Design review of the part built by this model. Coordinates are the model's own, in mm. Face numbers are marked on the shaded views. Coordinates: 2 decimals unless noted, no trailing zeros. Write each loop counter-clockwise with the first axis right and the second up, starting at its lowest first coordinate (ties: lowest second). Pieces come first, ordered by that corner, then holes. Notation, with made-up numbers: M -38.75,3.5 L -11.75,3.5 A20 ccw -11.75,13.5 Z; hole C -34.5,89.5 d8. An arc over 180 degrees is marked long. Write item = value, one per line.
```python
from build123d import *

# Parameters (mm, degrees)
F1_DEPTH = 53.975


with BuildPart() as f1:
    # F0 (on Right) → F1 (new body, symmetric)
    with BuildSketch(Plane.YZ):
        Polygon((-25.4, 14.664697), (-25.4, -14.664697), (0, -29.329394), (25.4, -14.664697), (25.4, 14.664697), (0, 29.329394), align=None)
    extrude(amount=F1_DEPTH, both=True)

    # F2 (on Front) → F3 (revolve, cut)
    with BuildSketch(Plane.XZ):
        Polygon((-53.975, 0), (53.975, 0), (53.975, 12.192), (-26.401746, 12.192), (-53.975, 20.543119), align=None)
    revolve(axis=Axis((-0.356656, 0, 0), (1, 0, 0)), mode=Mode.SUBTRACT)


solid = f1.part
```
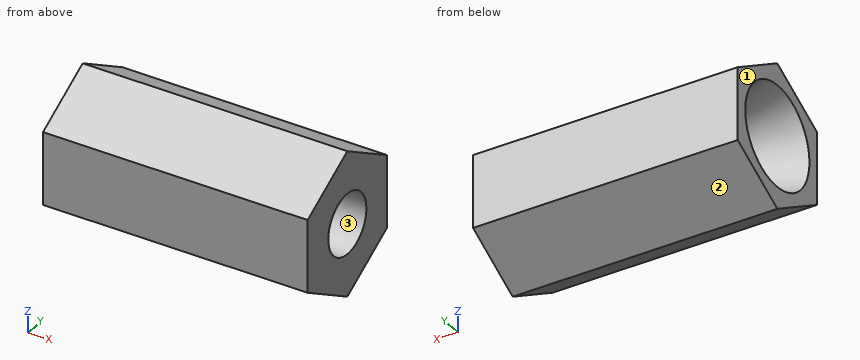
Q1. Consider section B-B, the plane z = 0. State the section outline as (x, y) points (3 decimals), and give its area (3 significant figures).
Check result:
outline = M -53.975,-25.4 L 53.975,-25.4 L 53.975,-12.192 L -26.402,-12.192 L -53.975,-20.543 Z; M -53.975,20.543 L -26.402,12.192 L 53.975,12.192 L 53.975,25.4 L -53.975,25.4 Z
area = 2,620 mm²
Q2. Consider section C-C, the plane z = -23.5. State the section outline as (x, y) points (3 decimals).
Check result:
outline = M -53.975,-10.097 L 53.975,-10.097 L 53.975,10.097 L -53.975,10.097 Z
Q3. Wall thickness on line 1 (Y direction, x = 25, z = 0); line 2 (Z direction, x = -9, y = 0); line 3 (Y direction, x = -37, z = -12): over which ranges is each line inside the solid? List them lowest first.
Check result:
line_1 = -25.4 to -12.19, 12.19 to 25.4
line_2 = -29.33 to -12.19, 12.19 to 29.33
line_3 = -25.4 to -9.65, 9.65 to 25.4
Q4. Consider section A-A, the plane x = 46.5. State the section outline as (y, z) points.
Check result:
outline = M -25.4,-14.66 L 0,-29.33 L 25.4,-14.66 L 25.4,14.66 L 0,29.33 L -25.4,14.66 Z; hole C 0,0 d24.38
Q5. The part is to be moulded in two halves that separate along Y. For the marked faces 1, 2 and 3, say which applies: +Y half, -Y half, draft (parallel to the pull), parting line (faces both ways), or undercut.
Check result:
face_1 = draft
face_2 = +Y half
face_3 = undercut
Q6. For P1, Ø1.5, axis at x = -37, y = 15, coming from the +Z side; P2, Ø1.5, axis at x = 38.5, z = -17, coming from the -Y side; P3, Ø10, axis at x = 5.5, y = -11, coming from the -Z side, all flat-tipped, find the tip position at first contact; note any pin that passes through.
Check result:
P1 = 21.1
P2 = -22.65
P3 = -25.87
